Geometry check sheet. Reference: drawing and pictorial views, mm from the part's lowest x, y, z. A direction names the side the tool comes from. Coordinates: 2 decimals unless noted, no trailing zeros. Loops run counter-clockwise (first coordinate to the right, second up) from the corner with the lowest first, then second, coordinate; pieces in that order, holes last. Notation, with made-up numbers: (-3.5, 61.5) - (38.5, 61.5) arc R12 ccw to (38.5, 77.5) - close; hole circle Ø11 at (-29.5, 87.25). An arc over 180 degrees is marked (long way). Use a Markdown table: item, result. Add a question column.
1) Tool access check on the marked faces 4 and 5. Record the directions out of +Z, -Z, +X, -X, +Y, -Y that give a thin tool (end or side, any length) a straight path to the whole face; none if there is none.
2) Sectioned sample at A-A, the plane y = 6. Enter the section's corners in (x, z).
3) Sectioned sample at D-D, the plane z = 12.5. Enter the section's corners in (x, y).
4) Go/stop test with flat-tipped pins: P1, Ø1.5, axis at x = 2, y = 52.5, coming from the -Z side; P2, Ø4, axis at x = 8.5, z = 53, coming from the +Y side; P3, Ø1, axis at x = 3.5, y = 46.5, coming from the +Z side. Record where each tip stops, or that it passes through.
5) Thickness scan on line 1 (Z direction, x = 6.75, y = 33); line 2 (Y direction, x = 4.75, z = 30.5); line 3 (Y direction, x = 8.5, z = 31.5). Record the ranges inside material, lowest first.
6) Sectioned sample at C-C, the plane x = 11.5. Enter the section's corners in (y, z) (3 decimals).
7) Draft check along Z on the marked faces 1, 2 and 3. Enter one of: pulls with the +Z half, pulls with the -Z half, needs draft (parallel to the pull), parting line crosses it, or undercut.
8) Sectioned sample at B-B, the plane z = 38.5. Enter the section's corners in (x, y), then the cut area to 3 significant figures.
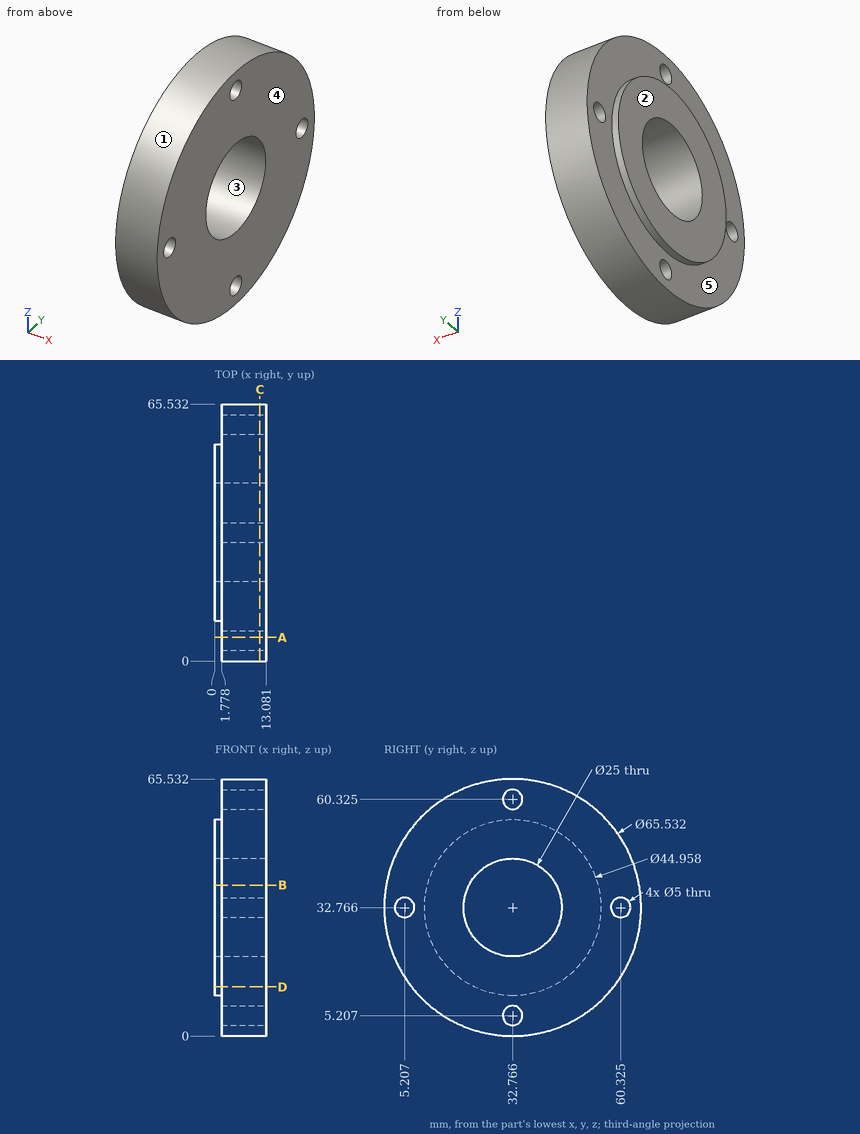
Solved:
| question | item | result |
|---|---|---|
| 1 | face 4 | +Z, -Z, +X, +Y, -Y |
| 1 | face 5 | -X |
| 2 | outline | (1.78, 13.87) - (13.08, 13.87) - (13.08, 30.4) - (1.78, 30.4) - close; (1.78, 35.14) - (13.08, 35.14) - (13.08, 51.67) - (1.78, 51.67) - close |
| 3 | outline | (0, 23.04) - (1.78, 23.04) - (1.78, 7.02) - (13.08, 7.02) - (13.08, 58.51) - (1.78, 58.51) - (1.78, 42.49) - (0, 42.49) - close |
| 4 | P1 | stops at z = 6.06 |
| 4 | P2 | stops at y = 59.99 |
| 4 | P3 | stops at z = 62.74 |
| 5 | line 1 | z = 0 to 2.72, 7.7 to 20.27, 45.26 to 57.84, 62.81 to 65.53 |
| 5 | line 2 | y = 0.08 to 4.15, 6.26 to 20.47, 45.06 to 59.27, 61.38 to 65.45 |
| 5 | line 3 | y = 0.02 to 3.05, 7.36 to 20.33, 45.2 to 58.17, 62.48 to 65.51 |
| 6 | outline | circle Ø65.532 at (32.766, 32.766); hole circle Ø5 at (5.207, 32.766); hole circle Ø25 at (32.766, 32.766); hole circle Ø5 at (32.766, 5.207); hole circle Ø5 at (32.766, 60.325); hole circle Ø5 at (60.325, 32.766) |
| 7 | face 1 | parting line crosses it |
| 7 | face 2 | needs draft |
| 7 | face 3 | undercut |
| 8 | outline | (0, 11.03) - (1.78, 11.03) - (1.78, 0.51) - (13.08, 0.51) - (13.08, 21.66) - (0, 21.66) - close; (0, 43.87) - (13.08, 43.87) - (13.08, 65.03) - (1.78, 65.03) - (1.78, 54.5) - (0, 54.5) - close |
| 8 | area | 516 mm2 |
